Part model, mm, in its own coordinate system. A direction names the side the tool comes from. Give positions to 0.01 mm unless a question says otherwise; leave off trailing zeros. Write each loop counter-clockwise with the first axis right and the second up, starting at its lowest first coordinate (ties: lowest second). Pieces come first, ordered by that corner, then holes.
from build123d import *

# Parameters (mm, degrees)
MODEL_R             = 14.351
MODEL_R_2           = 2.413
BOSS_EXTRUDE1_DEPTH = 6.35


with BuildPart() as part:
    # Model → Boss-Extrude1 (new body)
    with BuildSketch(Plane.XY):
        with BuildLine():
            ThreePointArc((-212.899365952, 93.541257838), (-203.778989185, 101.701881024), (-191.901103209, 104.650248016))
            Line((-191.901103209, 104.650248016), (48.661197018, 104.650248016))
            ThreePointArc((48.661197018, 104.650248016), (64.032332507, 99.471232012), (73.135172194, 86.046168785))
            Line((73.135172194, 86.046168785), (86.727013732, 37.098218434))
            ThreePointArc((86.727013732, 37.098218434), (106.36258142, 15.501750179), (127.326236921, 35.811553418))
            Line((127.326236921, 35.811553418), (140.807890588, 110.809453484))
            ThreePointArc((140.807890588, 110.809453484), (138.675228362, 126.361225539), (127.809114585, 137.689660276))
            Line((127.809114585, 137.689660276), (-44.466784077, 230.040741354))
            Line((-44.466784077, 230.040741354), (-154.507929168, 289.02994873))
            Line((-154.507929168, 289.02994873), (-199.949582693, 313.389629113))
            ThreePointArc((-199.949582693, 313.389629113), (-219.402189514, 318.224062751), (-236.303247901, 307.447705012))
            Line((-236.303247901, 307.447705012), (-425.920878295, 28.83612519))
            ThreePointArc((-425.920878295, 28.83612519), (-430.307847502, 13.679090678), (-424.898106806, -1.143726181))
            Line((-424.898106806, -1.143726181), (-385.58146606, -51.20282143))
            ThreePointArc((-385.58146606, -51.20282143), (-376.71145599, -58.357541068), (-365.605974805, -60.913979882))
            Line((-365.605974805, -60.913979882), (-324.737451002, -60.913979882))
            ThreePointArc((-324.737451002, -60.913979882), (-318.798508014, -59.439796386), (-314.23831963, -55.359484793))
            Line((-314.23831963, -55.359484793), (-212.899365952, 93.541257838))
        make_face()
        with Locations((-323.775189267, -35.513979882)):
            Circle(MODEL_R, mode=Mode.SUBTRACT)
        with Locations((-399.975189267, 2.586020118)):
            Circle(MODEL_R, mode=Mode.SUBTRACT)
        with Locations((107.189078625, 23.111553418)):
            Circle(MODEL_R_2, mode=Mode.SUBTRACT)
        with Locations((94.306236921, 35.628711714)):
            Circle(MODEL_R_2, mode=Mode.SUBTRACT)
        Polygon((110.67241113, 42.161553418), (114.338585339, 35.811553418), (110.67241113, 29.461553418), (103.340062711, 29.461553418), (99.673888502, 35.811553418), (103.340062711, 42.161553418), (106.823395217, 42.161553418), align=None, mode=Mode.SUBTRACT)
        with Locations((119.706236921, 35.994395122)):
            Circle(MODEL_R_2, mode=Mode.SUBTRACT)
        with Locations((106.823395217, 48.511553418)):
            Circle(MODEL_R_2, mode=Mode.SUBTRACT)
        with Locations((-190.707148919, 138.516914683)):
            Circle(MODEL_R, mode=Mode.SUBTRACT)
        with Locations((-175.899669139, 268.100247422)):
            Circle(MODEL_R_2, mode=Mode.SUBTRACT)
        with Locations((-208.832932893, 283.437784316)):
            Circle(MODEL_R, mode=Mode.SUBTRACT)
        with Locations((-166.899276125, 284.889989099)):
            Circle(MODEL_R_2, mode=Mode.SUBTRACT)
        with Locations((-51.007069668, 217.840195735)):
            Circle(MODEL_R_2, mode=Mode.SUBTRACT)
        with Locations((-31.957069668, 217.840195735)):
            Circle(MODEL_R_2, mode=Mode.SUBTRACT)
    extrude(amount=BOSS_EXTRUDE1_DEPTH)


solid = part.part
1) Saw through at B-B (x = 36). Write the cut outline in (y, z), and give its area (3 significant figures).
Check result:
outline: (104.65, 0) - (186.91, 0) - (186.91, 6.35) - (104.65, 6.35) - close
area: 522 mm2
2) Mould opens along Y. For faces 3 (the flat face through (-329.785, 170.092, 3.131)), 4 (the cylindrical face through (-177.45, 133.02, 3.13)), 5 (the flat face through (-405.515, -25.823, 3.131)) say: +Y half, -Y half, draft (parallel to the pull), parting line (faces both ways), or undercut.
Check result:
face 3: +Y half
face 4: undercut
face 5: -Y half
3) Saw through at A-A (y = 67). Write the cut outline in (x, z).
Check result:
outline: (-399.95, 0) - (-230.96, 0) - (-230.96, 6.35) - (-399.95, 6.35) - close; (78.42, 0) - (132.93, 0) - (132.93, 6.35) - (78.42, 6.35) - close
4) Flat gauge pins, fed straight in: P1, Ø3, axis at x = -175.9, y = 268.1, coming from the -Z side; P2, Ø7.5, axis at x = 107.19, y = 23.11, coming from the -Z side; P3, Ø1.5, axis at y = 35.5, z = 4.5, coming from the -X side; P4, Ø3, axis at x = -30.5, z = 1.5, coming from the -Y side. Where does each tip first touch, or does it go through?
Check result:
P1: passes through
P2: stops at z = 0
P3: stops at x = -421.9
P4: stops at y = 104.65
5) Saw through at C-C (z = 1.75). State how many separate pieces and enclosed holes the cut face has, and give its area (3 significant figures).
Check result:
separate pieces: 1
enclosed holes: 13
area: 87,200 mm2
6) Saw through at D-D (y = 248). Write the cut outline in (x, z), and give its area (3 significant figures).
Check result:
outline: (-276.76, 0) - (-77.97, 0) - (-77.97, 6.35) - (-276.76, 6.35) - close
area: 1,260 mm2
7) 3-axis set-ups, long thin cutter, end or side, ignore diameter. For faces 1 (the cylindrical face through (63.85, 99.61, 3.13)), 2 (the cylindrical face through (-210.701, 297.667, 3.131)): which of +Z, -Z, +X, -X, +Y, -Y reach the whole face in a straight line?
Check result:
face 1: +Z, -Z, -Y
face 2: +Z, -Z
8) Drill centre lines: L1, parallel to Y at x = -202.5, z = 5.75; L2, parallel to X at y = 48.5, z = 0.5; L3, parallel to X at y = 40, z = 1.5. Where is each one in solid material? Low to high.
Check result:
L1: y = 102.33 to 130.34, 146.69 to 270.56, 296.32 to 315.09
L2: x = -412.54 to -243.55, 83.56 to 104.41, 109.24 to 129.61
L3: x = -418.32 to -249.34, 85.92 to 102.09, 111.92 to 128.08
